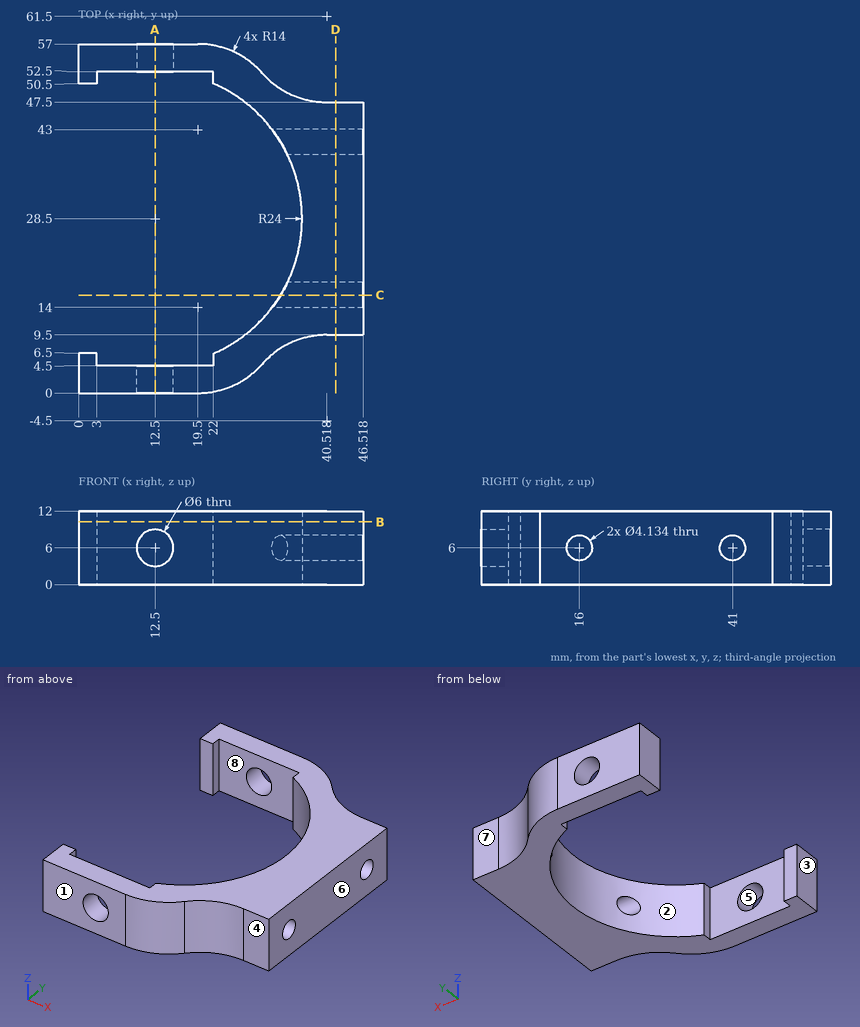
The drawing under review shows one solid part. Ordinate dimensions are in mm from its lowest x, y, z. A direction names the side the tool comes from. Give positions to 0.01 mm unless a question says otherwise; leave off trailing zeros. Order: outer loops, then holes, each group sorted by start corner. A loop starts at its lowest first (then second) coordinate and runs counter-clockwise, first axis right, second up. Notation, with made-up numbers: (9, 1) - (39, 1) arc R15 ccw to (39, 20) - close; hole circle Ø2 at (-33, 16). An arc over 180 degrees is marked (long way). Answer as a JSON object with one key per item and string values. Group by question number.
Item 1: Take a section at A-A on x = 12.5. Give the boundary of the cut face in (y, z), and give its area (3 significant figures).
Item 2: Take a section at C-C on y = 16. Give the boundary of the cut face in (x, z).
Item 3: Draft analysis for pull direction Y (two halves, no side actions). For the marked faces 1, 2 and 3, state which applies: pulls with the +Y half, pulls with the -Y half, needs draft (parallel to the pull), parting line crosses it, or undercut.
Item 4: Clearance check with flat-ended pins moving along their axes: pin 1 Ø1.6 at (y, z) = (51.5, 6) entering from +X; pin 2 Ø6.5 at (y, z) = (16, 6) entering from -X; pin 3 Ø1.8 at (x, z) = (44.5, 4.5) entering from -Y. State where each tip first meets the part, or that it passes through.
Item 5: Machinability: for the marked faces 4, 5, 6, 7 and 8, which of the approach directions +Z, -Z, +X, -X, +Y, -Y give a long, thin tool a straight path to every point of the face, cutting with its end or side? Answer none if there is none.
Item 6: Take a section at D-D on x = 42. Give the boundary of the cut face in (y, z).
Item 7: Take a section at B-B on z = 10.25. Give the boundary of the cut face in (x, y), and give its area (3 significant figures).
Item 8: Wall thickness on line 1 along Z through (x, y) = (41, 41); line 2 along Y through (x, z) = (3.5, 6.5); line 3 along Y through (x, z) = (41, 4.5): over which ranges is each line inside the solid? List them lowest first.
Reported:
{
 "1": {"outline": "(0, 0) - (4.5, 0) - (4.5, 3) - (0, 3) - close; (0, 9) - (4.5, 9) - (4.5, 12) - (0, 12) - close; (52.5, 0) - (57, 0) - (57, 3) - (52.5, 3) - close; (52.5, 9) - (57, 9) - (57, 12) - (52.5, 12) - close", "area": "54.0 mm^2"},
 "2": {"outline": "(32.99, 0) - (46.52, 0) - (46.52, 3.93) - (32.99, 3.93) - close; (32.99, 8.07) - (46.52, 8.07) - (46.52, 12) - (32.99, 12) - close"},
 "3": {"face 1": "pulls with the -Y half", "face 2": "undercut", "face 3": "needs draft"},
 "4": {"pin 1": "x = 31.61", "pin 2": "x = 30.61", "pin 3": "y = 9.5"},
 "5": {"face 4": "+Z, -Z, +X, -Y", "face 5": "+Y, -Y", "face 6": "+Z, -Z, +X, +Y, -Y", "face 7": "+Z, -Z, +X, +Y", "face 8": "+Z, -Z"},
 "6": {"outline": "(9.5, 0) - (47.5, 0) - (47.5, 12) - (9.5, 12) - close; hole circle Ø4.13 at (16, 6); hole circle Ø4.13 at (41, 6)"},
 "7": {"outline": "(0, 0) - (19.5, 0) arc R14 ccw to (30.01, 4.75) arc R14 cw to (40.52, 9.5) - (46.52, 9.5) - (46.52, 47.5) - (40.52, 47.5) arc R14 cw to (30.01, 52.25) arc R14 ccw to (19.5, 57) - (0, 57) - (0, 50.5) - (3, 50.5) - (3, 52.5) - (22, 52.5) - (22, 50.54) arc R24 cw to (22, 6.46) - (22, 4.5) - (3, 4.5) - (3, 6.5) - (0, 6.5) - close", "area": "833 mm^2"},
 "8": {"line 1": "0 to 3.93, 8.07 to 12", "line 2": "0 to 4.5, 52.5 to 57", "line 3": "9.5 to 14.58, 17.42 to 39.58, 42.42 to 47.5"}
}
